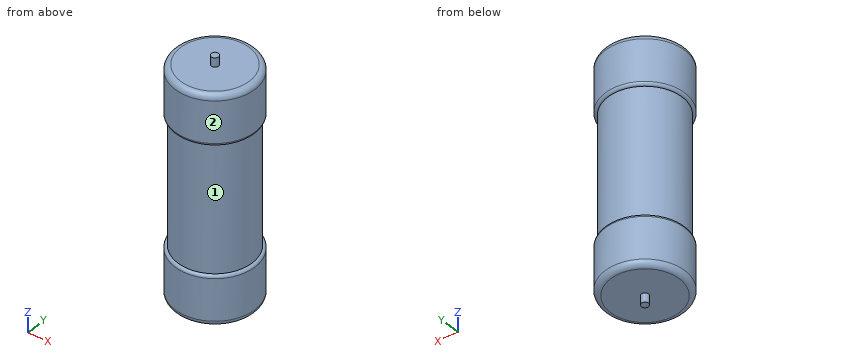
Autodesk Inventor part; units mm, degrees
ref_plane "YZ Plane" through (0, 0, 0) normal (1, 0, 0) x (0, 1, 0)
ref_plane "XZ Plane" through (0, 0, 0) normal (0, 1, 0) x (-1, 0, 0)
ref_plane "XY Plane" through (0, 0, 0) normal (0, 0, 1) x (1, 0, 0)
sketch "Skizze1" plane through (0, 0, 0) normal (0, 0, 1) x (1, 0, 0)
  circle A0 centre (0, 0) radius 4.4
  dimension "d0" = 8.8
extrude "Extrusion1" add sketch "Skizze1" along normal mid plane 25
sketch "Skizze4" plane through (0, 0, 0) normal (0, 0, 1) x (1, 0, 0)
  circle A0 centre (0, 0) radius 4.4
  circle A1 centre (0, 0) radius 4.1
  dimension "d10" = 0.3
extrude "Extrusion4" cut sketch "Skizze4" along normal mid plane 14
fillet "Rundung1" radius 0.3 2 edges at (-4.4, 0, 7) (-4.4, 0, -7)
fillet "Rundung2" radius 0.6 2 edges at (-4.4, 0, 12.5) (-4.4, 0, -12.5)
sketch "Skizze6" plane through (0, 0, 12.5) normal (0, 0, 1) x (1, 0, 0)
  circle A0 centre (0, 0) radius 0.405
  dimension "d21" = 0.81
extrude "Extrusion6" add sketch "Skizze6" along normal blind 1
mirror "Spiegeln3" about plane through (0, 0, 0) normal (0, 0, 1) of "Extrusion6"
properties part number "resistor WHS7 68R" material "Gummi, Silikon"
Geometry check sheet. Reference: the model listing, model coordinates, mm. Face numbers are marked on the shaded views. A direction names the side the tool comes from. Round coordinates to 2 decimals unless told otherwise and drop trailing zeros. Loops run counter-clockwise (first coordinate to the right, second up) from the corner with the lowest first, then second, coordinate; pieces in that order, holes last. Notation, with made-up numbers: (34, 83.5) - (74, 83.5) arc R19 ccw to (74, 105.5) - close; hole circle Ø5 at (64.25, 69). An arc over 180 degrees is marked (long way). Write each question's results on one line, items separated by ' | '. Start each with the question number.
Q1. Thickness scan on line 1 (Z direction, x = 3, y = 1); line 2 (Y direction, x = -0.75, z = 5.5); line 3 (X direction, y = 3, z = -3). Record the ranges inside material, lowest first. Write a range as [from, to].
Q2. Cross-section at C-C on z = 8.5. Enter the section's corners in (x, y), and give its area (3 significant figures).
Q3. Gauge pin test, flat ends, axial feed: P1, Ø3, axis at y = -3.5, z = 6.5, coming from the -X side; P2, Ø4, axis at y = -3, z = -9, coming from the +X side; P3, Ø5, axis at x = 3, z = 7.5, coming from the -Y side. Record the tip position at first contact, or that the pin passes through.
Q4. Cross-section at D-D on z = 1. Enter the section's corners in (x, y).
Q5. Access from +Z, -Z, +X, -X, +Y, -Y to the whole of each face (thin tool, end or side, straight path). Record for the marked faces 1 and 2.
Answers below:
1) line 1: z = [-12.5, 12.5] | line 2: y = [-4.03, 4.03] | line 3: x = [-2.79, 2.79]
2) outline: circle Ø8.8 at (0, 0) | area: 60.8 mm²
3) P1: stops at x = -3.81 | P2: stops at x = 4.28 | P3: stops at y = -4.37
4) outline: circle Ø8.2 at (0, 0)
5) face 1: none | face 2: +Z, -Z
